Design review of the part built by this model. Coordinates are the model's own, in mm. A direction names the side the tool comes from. Round coordinates to 2 decimals unless told otherwise and drop trailing zeros. Loops run counter-clockwise (first coordinate to the right, second up) from the corner with the lowest first, then second, coordinate; pieces in that order, holes last. Notation, with made-up numbers: (-9, 1.25) -> (6, 1.25) arc R15 ccw to (6, 14.25) -> close; hole circle Ø10 at (-22.75, 82). An arc over 180 degrees is marked (long way). Write each question's results on one line, items separated by ' | '. Start each with the question number.
from build123d import *

# Parameters (mm, degrees)
EXTRUDE_1_DEPTH     = 42.5
SKETCH_2_OUTSIDE_W  = 111.162
SKETCH_2_OUTSIDE_H  = 38.162
CUT_EXTRUDE_1_DEPTH = 86
SKETCH_3_W          = 52
SKETCH_3_H          = 52
CUT_EXTRUDE_2_DEPTH = 13
SKETCH_4_W          = 82
SKETCH_4_H          = 82
CUT_EXTRUDE_3_DEPTH = 2


with BuildPart() as part:
    # Эскиз1 → Бобышка-Вытянуть1 (new body, symmetric)
    with BuildSketch(Plane.XY):
        Polygon((0, 0), (-85, 0), (-85, 4), (-70, 12), (-15, 12), (0, 4), align=None)
    extrude(amount=EXTRUDE_1_DEPTH, both=True)

    # Эскиз2 outside → Вырез-Вытянуть1 (cut, through all)
    with BuildSketch(Plane(origin=(0, 0, 0), x_dir=(0, 0, -1), z_dir=(1, 0, 0))):
        with Locations((0, 6)):
            Rectangle(SKETCH_2_OUTSIDE_W, SKETCH_2_OUTSIDE_H)
        Polygon((-42.5, 4), (-42.5, 0), (42.5, 0), (42.5, 4), (27.5, 12), (-27.5, 12), align=None, mode=Mode.SUBTRACT)
    extrude(amount=-CUT_EXTRUDE_1_DEPTH, mode=Mode.SUBTRACT)

    # Эскиз3 → Вырез-Вытянуть2 (cut, through all)
    with BuildSketch(Plane.XZ):
        with Locations((-42.5, 0)):
            Rectangle(SKETCH_3_W, SKETCH_3_H)
    extrude(amount=-CUT_EXTRUDE_2_DEPTH, mode=Mode.SUBTRACT)

    # Эскиз4 → Вырез-Вытянуть3 (cut)
    with BuildSketch(Plane.XZ):
        with Locations((-42.5, 0)):
            Rectangle(SKETCH_4_W, SKETCH_4_H)
    extrude(amount=-CUT_EXTRUDE_3_DEPTH, mode=Mode.SUBTRACT)


solid = part.part
1) To check wall thickness, follow line 1 (X direction, y = 0.75, z = 13); line 2 (Y direction, x = -70, z = -11); line 3 (X direction, y = 2.5, z = 25). State the ranges of each line that lie inside material, in increasing order. Write a range as from..to.
2) Take a section at C-C (y = 5.5). Write out the cut boundary in (x, z).
3) Take a section at A-A (x = -50.5). Write out the cut boundary in (y, z), plus the area to 3 significant figures.
4) The part is to be moulded in two halves that separate along X. For faces 1 (the face through (-77.605, 7.944, 0.595)), 2 (the face through (-7.605, 8.056, 0.595)), 3 (the face through (-44.7, 12, -26.4)), 4 (the face through (-1.5, 1, -1)), say which applies: +X half, -X half, draft (parallel to the pull), parting line (faces both ways), or undercut.
5) Take a section at D-D (z = 36.5). Write out the cut boundary in (x, y), plus the area to 3 significant figures.
6) For faces 5 (the face through (-43, 1, 41)), 6 (the face through (-43, 7, 26)), 7 (the face through (-42, 2, -42.5)), list the 3-axis set-ups (+Z, -Z, +X, -X, +Y, -Y) from which the entire face can be reached by the end or side of a thin tool; tool diameter is ignored.
7) Insertion check: pin 1 (0.6 mm diameter, centred on y = 1, z = -11, fed in from +X); pin 2 (6 mm diameter, centred on x = -47.5, y = 10, fed in from +Z) (3 decimals); pin 3 (10 mm diameter, centred on x = -43.5, z = 28.5, fed in from -Y); pin 4 (3 mm diameter, centred on y = 8.5, z = 3, fed in from -X) (3 decimals). Each pin has a flat end and moves straight along its axis. Give the tip position at first contact, or say it passes through.
8) Take a section at B-B (z = -24). Write out the cut boundary in (x, y), plus the area to 3 significant figures.
Geometry check:
1) line 1: x = -85..-83.5, -1.5..0 | line 2: y = 2..12 | line 3: x = -85..-68.5, -16.5..0
2) outline: (-82.19, -39.69) -> (-2.81, -39.69) -> (-2.81, 39.69) -> (-82.19, 39.69) -> close; hole (-68.5, -26) -> (-16.5, -26) -> (-16.5, 26) -> (-68.5, 26) -> close
3) outline: (0, -42.5) -> (4, -42.5) -> (12, -27.5) -> (12, -26) -> (2, -26) -> (2, -41) -> (0, -41) -> close; (0, 41) -> (2, 41) -> (2, 26) -> (12, 26) -> (12, 27.5) -> (4, 42.5) -> (0, 42.5) -> close | area: 216 mm^2
4) face 1: -X half | face 2: +X half | face 3: draft | face 4: undercut
5) outline: (-85, 0) -> (-83.5, 0) -> (-83.5, 2) -> (-1.5, 2) -> (-1.5, 0) -> (0, 0) -> (0, 4) -> (-6, 7.2) -> (-79, 7.2) -> (-85, 4) -> close | area: 429 mm^2
6) face 5: -Y | face 6: +Y, -Y | face 7: -Z, +X, -X, +Y, -Y
7) pin 1: stops at x = 0 | pin 2: stops at z = 36.875 | pin 3: stops at y = 2 | pin 4: stops at x = -79.375
8) outline: (-85, 0) -> (-83.5, 0) -> (-83.5, 2) -> (-68.5, 2) -> (-68.5, 12) -> (-70, 12) -> (-85, 4) -> close; (-16.5, 2) -> (-1.5, 2) -> (-1.5, 0) -> (0, 0) -> (0, 4) -> (-15, 12) -> (-16.5, 12) -> close | area: 216 mm^2
